For this review, take the finished solid that the model builds, in its own axes (mm). Coordinates: 2 decimals unless noted, no trailing zeros. Order: outer loops, then holes, each group sorted by start corner. A loop starts at its lowest first (then second) coordinate and runs counter-clockwise, first axis right, second up. Notation, with made-up numbers: (52.25, 49) - (93.25, 49) arc R27 ccw to (93.25, 73) - close; hole circle Ø4 at (-26.75, 89.25). An arc over 180 degrees is marked (long way). One line per item, written item: value. Start each with the question number.
(1) To check wall thickness, follow line 1 along Z through (x, y) = (-6.75, 31.25); line 2 along Z through (x, y) = (-11.5, 39.5); line 3 along X through (y, z) = (36.5, -2). State the ranges of each line that lie inside material, in increasing order.
(2) Consider section A-A on y = 38. Write out the cut boundary in (x, z), then the cut area to 3 significant figures.
(3) Consider section C-C on z = -4.25. Write out the cut boundary in (x, y).
(4) Clearance check with flat-ended pins moving along their axes: pin 1 (1.5 mm diameter, centred on y = 29.5, z = -19, fed in from +X); pin 2 (3 mm diameter, centred on x = -10, y = 30.5, fed in from +Z). State where each tip first meets the part, or that it passes through.
(5) Consider section B-B on x = -14.75. Write out the cut boundary in (y, z).
```python
from build123d import *

# Parameters (mm, degrees)
SKETCH023_W     = 16
SKETCH023_H     = 16
PAD013_DEPTH    = 28.8
POCKET010_DEPTH = 16
POCKET047_DEPTH = 16
PAD140_DEPTH    = 16


with BuildPart() as part:
    # Sketch023 (on Face56 of Binder009) → Pad013 (new body)
    with BuildSketch(Plane.XY.offset(-28.8)):
        with Locations((-8, 32)):
            Rectangle(SKETCH023_W, SKETCH023_H)
    extrude(amount=PAD013_DEPTH)

    # Sketch024 (on Face3 of Pad013) → Pocket010 (cut)
    with BuildSketch(Plane.XZ.offset(-24)):
        Polygon((-16, -9.6), (0, 0), (-16, 0), align=None)
    extrude(amount=-POCKET010_DEPTH, mode=Mode.SUBTRACT)

    # Sketch138 (on Face6 of Pocket010) → Pocket047 (cut)
    with BuildSketch(Plane.XZ.offset(-24)):
        Polygon((0, 0), (-3.2, 0), (-16, -7.68), (-16, -10.88), (-3.2, -3.2), (0, -3.2), align=None)
    extrude(amount=-POCKET047_DEPTH, mode=Mode.SUBTRACT)

    # Sketch138 (on Face6 of Pocket010) → Pad140 (join)
    with BuildSketch(Plane.XZ.offset(-24)):
        Polygon((0, 0), (-3.2, 0), (-16, -7.68), (-16, -10.88), (-3.2, -3.2), (0, -3.2), align=None)
    extrude(amount=-PAD140_DEPTH)


solid = part.part
```
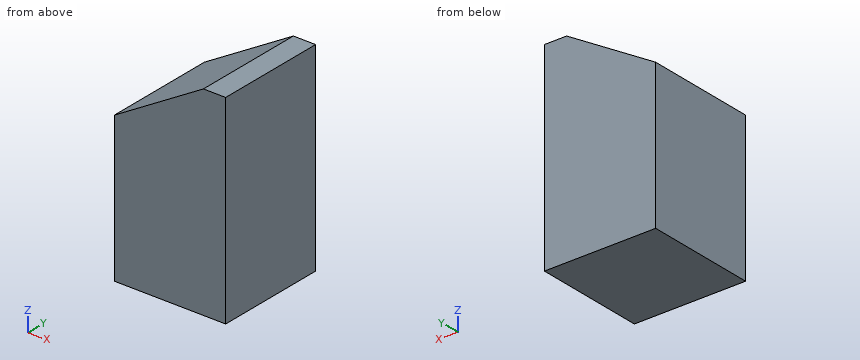
Geometry check:
1. line 1: z = -28.8 to -2.13
1. line 2: z = -28.8 to -4.98
1. line 3: x = -6.53 to 0
2. outline: (-16, -28.8) - (0, -28.8) - (0, 0) - (-3.2, 0) - (-16, -7.68) - close
2. area: 412 mm^2
3. outline: (-10.28, 24) - (0, 24) - (0, 40) - (-10.28, 40) - close
4. pin 1: stops at x = 0
4. pin 2: stops at z = -3.18
5. outline: (24, -28.8) - (40, -28.8) - (40, -6.93) - (24, -6.93) - close
